Design review of the part built by this model. Coordinates are the model's own, in mm. A direction names the side the tool comes from. Round coordinates to 2 decimals unless told otherwise and drop trailing zeros. Order: outer loops, then holes, each group sorted by start corner. A loop starts at its lowest first (then second) coordinate and runs counter-clockwise, first axis right, second up.
from build123d import *


with BuildPart() as part:
    # Sketch1 → Revolve1 (revolve)
    with BuildSketch(Plane(origin=(0, 0, 0), x_dir=(0, 0, -1), z_dir=(1, 0, 0)), mode=Mode.PRIVATE) as revolve1_sk:
        with BuildLine():
            Line((-1.5, -1.95), (-1.5, 1.95))
            Line((-1.5, 1.95), (-3.25, 1.95))
            ThreePointArc((-3.25, 1.95), (-3.780330086, 1.730330086), (-4, 1.2))
            Line((-4, 1.2), (-4, 0.75))
            Line((-4, 0.75), (-3, 0.75))
            Line((-3, 0.75), (-3, -0.75))
            Line((-3, -0.75), (-4, -0.75))
            Line((-4, -0.75), (-4, -1.2))
            ThreePointArc((-4, -1.2), (-3.780330086, -1.730330086), (-3.25, -1.95))
            Line((-3.25, -1.95), (-1.5, -1.95))
        make_face()
    revolve(revolve1_sk.sketch.rotate(Axis((0, 0, 0), (0, 1, 0)), 180), axis=Axis((0, 0, 0), (0, 1, 0)))


solid = part.part
1) Take a section at A-A on z = 0. Give the boundary of the cut face in (x, y), plus the area to 3 significant figures.
Results:
outline: (-4, -1.2) arc R0.75 ccw to (-3.25, -1.95) - (-1.5, -1.95) - (-1.5, 1.95) - (-3.25, 1.95) arc R0.75 ccw to (-4, 1.2) - (-4, 0.75) - (-3, 0.75) - (-3, -0.75) - (-4, -0.75) - close; (1.5, -1.95) - (3.25, -1.95) arc R0.75 ccw to (4, -1.2) - (4, -0.75) - (3, -0.75) - (3, 0.75) - (4, 0.75) - (4, 1.2) arc R0.75 ccw to (3.25, 1.95) - (1.5, 1.95) - close
area: 16.0 mm2
2) For faces 1 (the face through (-0.9, -0.01, -2.86)), 2 (the face through (-1.5, -1.95, -0.7)), list the 3-axis set-ups (+Z, -Z, +X, -X, +Y, -Y) from which the entire face can be reached by the end or side of a thin tool; tool diameter is ignored.
Results:
face 1: none
face 2: +Z, -Z, +X, -X, -Y
3) Take a section at B-B on x = 0. Give the boundary of the cut face in (y, z).
Results:
outline: (-1.95, -3.25) arc R0.75 ccw to (-1.2, -4) - (-0.75, -4) - (-0.75, -3) - (0.75, -3) - (0.75, -4) - (1.2, -4) arc R0.75 ccw to (1.95, -3.25) - (1.95, -1.5) - (-1.95, -1.5) - close; (-1.95, 1.5) - (1.95, 1.5) - (1.95, 3.25) arc R0.75 ccw to (1.2, 4) - (0.75, 4) - (0.75, 3) - (-0.75, 3) - (-0.75, 4) - (-1.2, 4) arc R0.75 ccw to (-1.95, 3.25) - close
4) To check wall thickness, follow line 1 along X through (y, z) = (0.6, 0); line 2 along X through (y, z) = (-1, 0); line 3 along Y through (x, z) = (-2.75, -1.75). State the ranges of each line that lie inside material, in increasing order.
Results:
line 1: x = -3 to -1.5, 1.5 to 3
line 2: x = -4 to -1.5, 1.5 to 4
line 3: y = -1.95 to -0.75, 0.75 to 1.95
5) Take a section at D-D on y = -0.4. Give the boundary of the cut face in (x, z), plus the area to 3 significant figures.
Results:
outline: circle Ø6 at (0, 0); hole circle Ø3 at (0, 0)
area: 21.2 mm2
6) Take a section at C-C on y = -0.95. Give the boundary of the cut face in (x, z).
Results:
outline: circle Ø8 at (0, 0); hole circle Ø3 at (0, 0)
7) The part is to be moulded in two halves that separate along Z. For faces 3 (the face through (-3, 0.75, -1)), 4 (the face through (3.905, -0.978, 0.867)), 5 (the face through (-0.45, 0.03, -1.43)), say which applies: released by +Z, released by -Z, zero draft, split by the parting line, or undercut.
Results:
face 3: zero draft
face 4: split by the parting line
face 5: undercut
8) Clearance check with a flat-ended pin moving along its axis: P1, Ø1.5, axis at x = 3, y = -0.5, coming from the -Z side. State where the tip first meets the part, or that it passes through.
Results:
P1: stops at z = -3.28
